Can you work these out from the drawing? Everything is in mm from the part's minimum corner. A direction names the side the tool comes from. Round coordinates to 2 decimals unless told otherwise and drop trailing zeros. Loops run counter-clockwise (first coordinate to the right, second up) from the corner with the lowest first, then second, coordinate; pieces in that order, holes last. Notation, with made-up numbers: M 2.5,69.25 L 20.5,69.25 A32 cw 20.5,101.25 Z; hole C 34,87 d9. An arc over 180 degrees is marked long. Use a Markdown table: item, result.
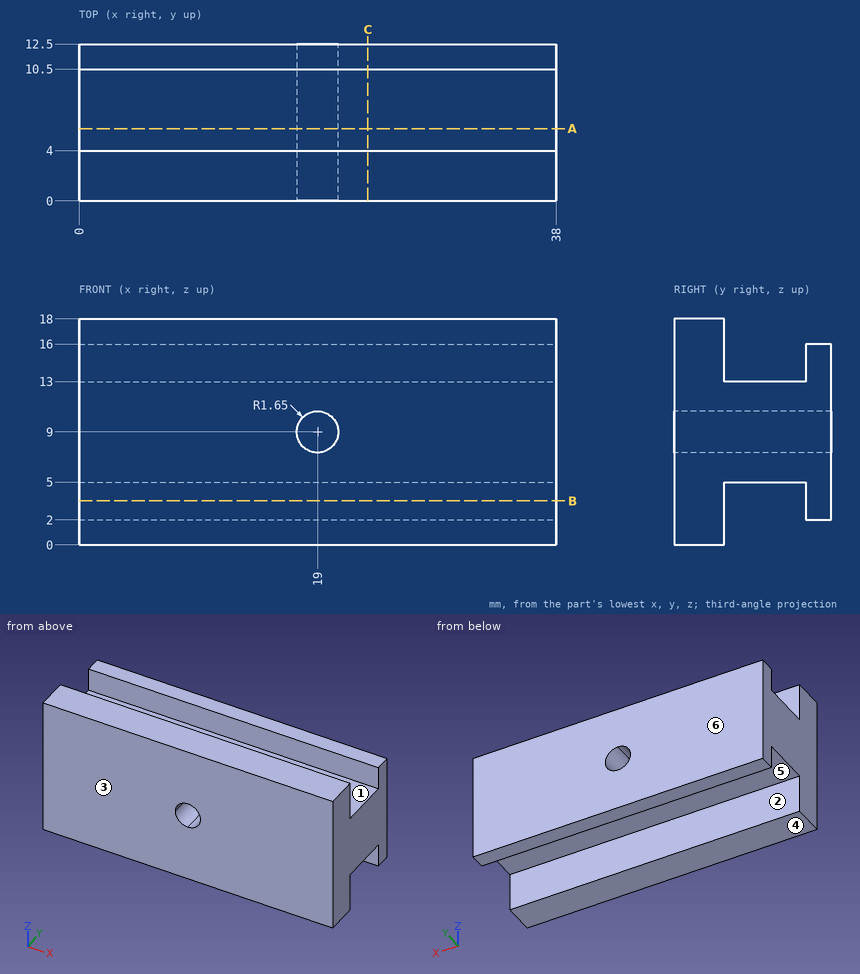
1. We'd pull the mould along Y, two halves only. Please class the marked faces 4, 5 and 6: +Y half, -Y half, draft (parallel to the pull), parting line (faces both ways), or undercut.
Answer sheet:
| item | result |
|---|---|
| face 4 | draft |
| face 5 | undercut |
| face 6 | +Y half |
2. I need wall thicknesses on probe 1 along Y at (x, z) = (24, 2.25); probe 2 along Z at (x, y) = (17, 5); probe 3 along X at (y, z) = (11.75, 9.25). Which ranges of each line are inside material? Lowest first, please. Write a range as from..to.
Answer sheet:
| item | result |
|---|---|
| probe 1 | 0..4, 10.5..12.5 |
| probe 2 | 5..13 |
| probe 3 | 0..17.37, 20.63..38 |
3. Imagine slicing it at A-A, the plane y = 5.75. Write out the boundary of the cut face in (x, z).
Answer sheet:
| item | result |
|---|---|
| outline | M 0,5 L 38,5 L 38,13 L 0,13 Z; hole C 19,9 d3.3 |
4. For pin 1 Ø2.5 at (x, z) = (10, 14) entering from -Y; pin 2 Ø4 at (x, y) = (7, 11) entering from -Z; pin 3 Ø2 at (x, y) = (24.5, 11.5) entering from +Z; pin 4 Ø3 at (x, y) = (34, 6.5) entering from +Z, each with a flat end and sliding along its axis, tell me the tip position at first contact or that it passes through.
Answer sheet:
| item | result |
|---|---|
| pin 1 | y = 0 |
| pin 2 | z = 2 |
| pin 3 | z = 16 |
| pin 4 | z = 13 |
5. Imagine slicing it at B-B, the plane z = 3.5. Write out the boundary of the cut face in (x, y).
Answer sheet:
| item | result |
|---|---|
| outline | M 0,0 L 38,0 L 38,4 L 0,4 Z; M 0,10.5 L 38,10.5 L 38,12.5 L 0,12.5 Z |
6. Imagine slicing it at C-C, the plane x = 23. Write out the boundary of the cut face in (y, z).
Answer sheet:
| item | result |
|---|---|
| outline | M 0,0 L 4,0 L 4,5 L 10.5,5 L 10.5,2 L 12.5,2 L 12.5,16 L 10.5,16 L 10.5,13 L 4,13 L 4,18 L 0,18 Z |
7. Which directions (+Z, -Z, +X, -X, +Y, -Y) give clear straight access to the entire face, cutting with the end or side of a thin tool? Please do the marked faces 1, 2 and 3.
Answer sheet:
| item | result |
|---|---|
| face 1 | +Z, +X, -X |
| face 2 | -Z, +X, -X |
| face 3 | +Z, -Z, +X, -X, -Y |
